Geometry check sheet. Reference: the model listing, model coordinates, mm. Face numbers are marked on the shaded views. A direction names the side the tool comes from. Coordinates: 2 decimals unless noted, no trailing zeros. Write each loop counter-clockwise with the first axis right and the second up, starting at its lowest first coordinate (ties: lowest second). Pieces come first, ordered by that corner, then holes. Notation, with made-up numbers: (47.25, -31) -> (60.25, -31) arc R29 cw to (60.25, 8) -> close; hole circle Ø5 at (-6, 47). An arc over 180 degrees is marked (long way). Answer in a Markdown table with one row per item. Add a question column.
1. Cross-section at B-B on y = 0. Record the cut outline in (x, z) (3 decimals).
2. Cross-section at A-A on x = -3.5. Record the cut outline in (y, z).
3. Cross-section at C-C on x = 0. Record the cut outline in (y, z) (3 decimals).
4. Set-up check for the marked faces 4, 5 and 6: record each of +Z, -Z, +X, -X, +Y, -Y from which the full face is reachable in a straight line by a thin tool's end or side.
5. Mould release check, pull along Y, two halves, no side actions. Record for the marked faces 1, 2 and 3: pulls with the +Y half, pulls with the -Y half, needs draft (parallel to the pull), parting line crosses it, or undercut.
6. Depth check by flat-ended pin: P1, Ø2, axis at y = 1, z = 29, coming from the -X side; P2, Ø4, axis at x = -1.5, z = 44, coming from the +Y side; P3, Ø2.5, axis at x = -1.5, z = 32, coming from the -Y side. Enter the tip coordinate at first touch or a pass-through.
7. Scan lines: L1, parallel to Y at x = 5.75, z = 24; L2, parallel to Z at x = 8, y = 7.75; L3, parallel to Z at x = -5, y = 2.5. Record each from-to range of solid material in increasing order. Write a range as from..to.
8. Cross-section at D-D on z = 23. Record the cut outline in (x, y) (3 decimals).
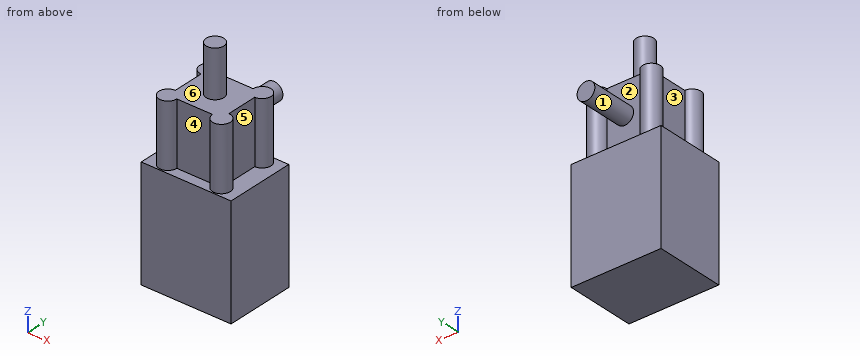
```python
from build123d import *

# Parameters (mm, degrees)
SKETCH1_W           = 20.11
SKETCH1_H           = 15.6
BOSS_EXTRUDE1_DEPTH = 24.91
SKETCH2_R           = 2
SKETCH2_W           = 12
SKETCH2_H           = 11
BOSS_EXTRUDE2_DEPTH = 14.05
SKETCH3_R           = 1.99
BOSS_EXTRUDE3_DEPTH = 10.45
SKETCH4_R           = 1.99
BOSS_EXTRUDE4_DEPTH = 10.48


with BuildPart() as part:
    # Sketch1 → Boss-Extrude1 (new body)
    with BuildSketch(Plane.XY):
        Rectangle(SKETCH1_W, SKETCH1_H)
    extrude(amount=BOSS_EXTRUDE1_DEPTH)

    # Sketch2 → Boss-Extrude2 (add)
    with BuildSketch(Plane.XY.offset(24.91)):
        with BuildLine():
            ThreePointArc((-4, 5.5), (-7.414213562, 6.914213562), (-6, 3.5))
            Line((-6, 3.5), (-6, 5.5))
            Line((-6, 5.5), (-4, 5.5))
        make_face()
        with BuildLine():
            Line((-6, 5.5), (-6, 3.5))
            ThreePointArc((-6, 3.5), (-4.585786438, 4.085786438), (-4, 5.5))
            Line((-4, 5.5), (-6, 5.5))
        make_face()
        with Locations((-6, -5.5)):
            Circle(SKETCH2_R)
        with Locations((6, -5.5)):
            Circle(SKETCH2_R)
        with Locations((6, 5.5)):
            Circle(SKETCH2_R)
        with Locations((-6, 5.5)):
            Circle(SKETCH2_R)
        Rectangle(SKETCH2_W, SKETCH2_H)
        with BuildLine():
            ThreePointArc((4, 5.5), (4.585786438, 4.085786438), (6, 3.5))
            Line((6, 3.5), (6, 5.5))
            Line((6, 5.5), (4, 5.5))
        make_face()
        with BuildLine():
            Line((6, 5.5), (6, 3.5))
            ThreePointArc((6, 3.5), (7.414213562, 4.085786438), (8, 5.5))
            ThreePointArc((8, 5.5), (6, 7.5), (4, 5.5))
            Line((4, 5.5), (6, 5.5))
        make_face()
        with BuildLine():
            ThreePointArc((6, -3.5), (4.585786438, -4.085786438), (4, -5.5))
            Line((4, -5.5), (6, -5.5))
            Line((6, -5.5), (6, -3.5))
        make_face()
        with BuildLine():
            Line((6, -5.5), (4, -5.5))
            ThreePointArc((4, -5.5), (6, -7.5), (8, -5.5))
            ThreePointArc((8, -5.5), (7.414213562, -4.085786438), (6, -3.5))
            Line((6, -3.5), (6, -5.5))
        make_face()
        with BuildLine():
            ThreePointArc((-6, -3.5), (-7.414213562, -6.914213562), (-4, -5.5))
            Line((-4, -5.5), (-6, -5.5))
            Line((-6, -5.5), (-6, -3.5))
        make_face()
        with BuildLine():
            Line((-6, -5.5), (-4, -5.5))
            ThreePointArc((-4, -5.5), (-4.585786438, -4.085786438), (-6, -3.5))
            Line((-6, -3.5), (-6, -5.5))
        make_face()
    extrude(amount=BOSS_EXTRUDE2_DEPTH)

    # Sketch3 → Boss-Extrude3 (add)
    with BuildSketch(Plane(origin=(0, 5.5, 0), x_dir=(1, 0, 0), z_dir=(0, 1, 0))):
        with Locations((0, -31.935)):
            Circle(SKETCH3_R)
    extrude(amount=BOSS_EXTRUDE3_DEPTH)

    # Sketch4 → Boss-Extrude4 (add)
    with BuildSketch(Plane.XY.offset(38.96)):
        with Locations(Location((0, 0, 0), (0, 0, 180))):
            Circle(SKETCH4_R)
    extrude(amount=BOSS_EXTRUDE4_DEPTH)


solid = part.part
```
Results found:
| question | item | result |
|---|---|---|
| 1 | outline | (-10.055, 0) -> (10.055, 0) -> (10.055, 24.91) -> (6, 24.91) -> (6, 38.96) -> (1.99, 38.96) -> (1.99, 49.44) -> (-1.99, 49.44) -> (-1.99, 38.96) -> (-6, 38.96) -> (-6, 24.91) -> (-10.055, 24.91) -> close |
| 2 | outline | (-7.8, 0) -> (7.8, 0) -> (7.8, 24.91) -> (5.5, 24.91) -> (5.5, 38.96) -> (-5.5, 38.96) -> (-5.5, 24.91) -> (-7.8, 24.91) -> close |
| 3 | outline | (-7.8, 0) -> (7.8, 0) -> (7.8, 24.91) -> (5.5, 24.91) -> (5.5, 29.945) -> (15.95, 29.945) -> (15.95, 33.925) -> (5.5, 33.925) -> (5.5, 38.96) -> (1.99, 38.96) -> (1.99, 49.44) -> (-1.99, 49.44) -> (-1.99, 38.96) -> (-5.5, 38.96) -> (-5.5, 24.91) -> (-7.8, 24.91) -> close |
| 4 | face 4 | +Z, -Y |
| 4 | face 5 | +Z, +X |
| 4 | face 6 | +Z |
| 5 | face 1 | needs draft |
| 5 | face 2 | pulls with the +Y half |
| 5 | face 3 | undercut |
| 6 | P1 | stops at x = -6 |
| 6 | P2 | stops at y = 1.99 |
| 6 | P3 | stops at y = -5.5 |
| 7 | L1 | y = -7.8..7.8 |
| 7 | L2 | z = 0..24.91 |
| 7 | L3 | z = 0..38.96 |
| 8 | outline | (-10.055, -7.8) -> (10.055, -7.8) -> (10.055, 7.8) -> (-10.055, 7.8) -> close |
